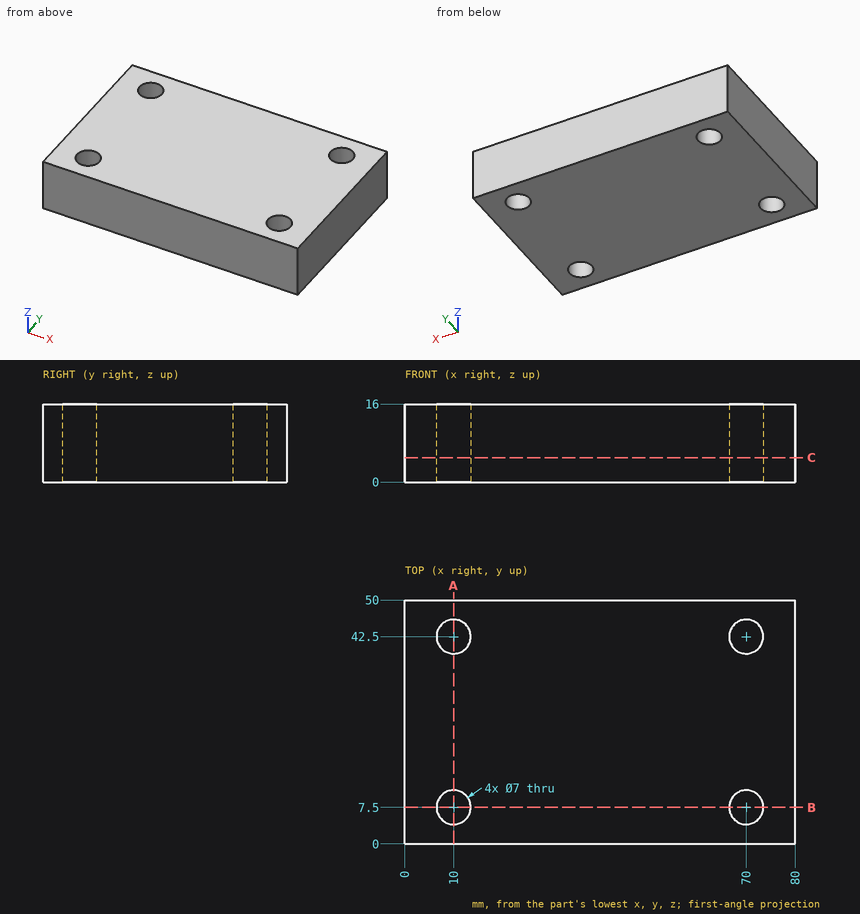
Study the drawing (mm; zero at the part's minimum x, y, z) and answer. Round coordinates to 2 decimals unless told otherwise and drop trailing zeros. Loops run counter-clockwise (first coordinate to the right, second up) from the corner with the lowest first, then second, coordinate; pieces in that order, holes last. Notation, with made-up numbers: (34.25, 12) -> (45.25, 12) arc R20 cw to (45.25, 16) -> close; hole circle Ø4 at (57.25, -15). An arc over 180 degrees is marked (long way). One line per item, written item: value.
1) A flat-ended cylindrical pin translates along its axis: P1, Ø5.5, axis at x = 70, y = 42.5, coming from the -Z side. Find the tip coordinate at first contact, or state that the pin passes through.
Answer list:
P1: passes through
2) A cutting plane is placed at B-B (y = 7.5). Determine the outline of the cut face in (x, z), and give its area (3 significant figures).
Answer list:
outline: (0, 0) -> (6.5, 0) -> (6.5, 16) -> (0, 16) -> close; (13.5, 0) -> (66.5, 0) -> (66.5, 16) -> (13.5, 16) -> close; (73.5, 0) -> (80, 0) -> (80, 16) -> (73.5, 16) -> close
area: 1,060 mm²
3) A cutting plane is placed at C-C (z = 5). Determine the outline of the cut face in (x, y), and give its area (3 significant figures).
Answer list:
outline: (0, 0) -> (80, 0) -> (80, 50) -> (0, 50) -> close; hole circle Ø7 at (10, 7.5); hole circle Ø7 at (10, 42.5); hole circle Ø7 at (70, 7.5); hole circle Ø7 at (70, 42.5)
area: 3,850 mm²
4) Consider L1, parallel to Y at x = 10, z = 12.75; L2, parallel to X at y = 43.5, z = 9.5; L3, parallel to X at y = 43, z = 11. Determine where each line is inside the solid, lowest interval first. Write a range as [from, to].
Answer list:
L1: y = [0, 4], [11, 39], [46, 50]
L2: x = [0, 6.65], [13.35, 66.65], [73.35, 80]
L3: x = [0, 6.54], [13.46, 66.54], [73.46, 80]
5) A cutting plane is placed at A-A (x = 10). Determine the outline of the cut face in (y, z).
Answer list:
outline: (0, 0) -> (4, 0) -> (4, 16) -> (0, 16) -> close; (11, 0) -> (39, 0) -> (39, 16) -> (11, 16) -> close; (46, 0) -> (50, 0) -> (50, 16) -> (46, 16) -> close
